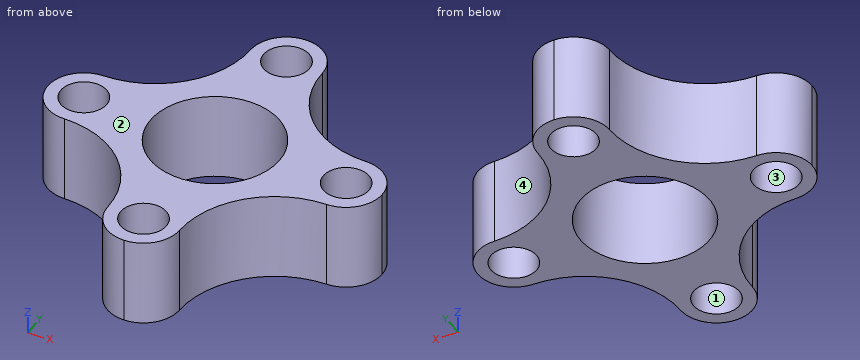
from build123d import *

# Parameters (mm, degrees)
AUFSATZ_LINEAR_AUSTRAGEN1_DEPTH = 10
SKIZZE2_R                       = 2.6
SCHNITT_LINEAR_AUSTRAGEN2_DEPTH = 10
SKIZZE3_R                       = 7.311453451
SCHNITT_LINEAR_AUSTRAGEN4_DEPTH = 10


with BuildPart() as part:
    # Skizze1 → Aufsatz-Linear austragen1 (new body)
    with BuildSketch(Plane.XY):
        with BuildLine():
            Line((0, 19.095775163), (0, 0))
            Line((0, 0), (19.095775163, 0))
            ThreePointArc((19.095775163, 0), (17.894912966, 2.899137803), (14.995775163, 4.1))
            ThreePointArc((14.995775163, 4.1), (7.291298659, 7.291298659), (4.1, 14.995775163))
            ThreePointArc((4.1, 14.995775163), (2.899137803, 17.894912966), (0, 19.095775163))
        make_face()
    extrude(amount=AUFSATZ_LINEAR_AUSTRAGEN1_DEPTH)

    # Spiegeln1: part across plane


with BuildPart() as part_1:
    add(part.part)
    add(part.part.mirror(Plane.ZX))

    # Spiegeln2: part across plane


with BuildPart() as part_2:
    add(part_1.part)
    add(part_1.part.mirror(Plane(origin=(0, 0, 0), x_dir=(0, 0, 1), z_dir=(1, 0, 0))))

    # Skizze2 → Schnitt-Linear austragen2 (cut)
    with BuildSketch(Plane.XY):
        with Locations((0, 14.995775163)):
            Circle(SKIZZE2_R)
        with Locations((14.995775163, 0)):
            Circle(SKIZZE2_R)
        with Locations((0, -14.995775163)):
            Circle(SKIZZE2_R)
        with Locations((-14.995775163, 0)):
            Circle(SKIZZE2_R)
    extrude(amount=SCHNITT_LINEAR_AUSTRAGEN2_DEPTH, mode=Mode.SUBTRACT)

    # Skizze3 → Schnitt-Linear austragen4 (cut)
    with BuildSketch(Plane.XY):
        Circle(SKIZZE3_R)
    extrude(amount=SCHNITT_LINEAR_AUSTRAGEN4_DEPTH, mode=Mode.SUBTRACT)


solid = part_2.part
Model file for the job. Use its own axes, mm. Face numbers are marked on the shaded views. Round coordinates to 2 decimals unless told otherwise and drop trailing zeros. Loops run counter-clockwise (first coordinate to the right, second up) from the corner with the lowest first, then second, coordinate; pieces in that order, holes last.
1. Drop flat-ended pins along their axis: P1, Ø1, axis at x = 2, z = 1.5, coming from the -Y side; P2, Ø2, axis at x = 8, z = 3.5, coming from the +Y side; P3, Ø1, axis at y = -2.5, z = 2, coming from the +X side. Give the stop position or say it passes through.
Check values:
P1: stops at y = -18.81
P2: stops at y = 7.59
P3: stops at x = 18.57
2. Band-saw the part on D-D, the plane y = 5.5. List the corners of the cut face in (x, z), and give its area (3 significant figures).
Check values:
outline: (-9.65, 0) - (-4.82, 0) - (-4.82, 10) - (-9.65, 10) - close; (4.82, 0) - (9.65, 0) - (9.65, 10) - (4.82, 10) - close
area: 96.7 mm2
3. Band-saw the part on B-B, the plane x = -14. List the corners of the cut face in (y, z), and give its area (3 significant figures).
Check values:
outline: (-4.15, 0) - (-2.4, 0) - (-2.4, 10) - (-4.15, 10) - close; (2.4, 0) - (4.15, 0) - (4.15, 10) - (2.4, 10) - close
area: 34.9 mm2
4. Band-saw the part on A-A, the plane z = 7.5. List the corners of the cut face in (x, y), and give its area (3 significant figures).
Check values:
outline: (-15, -4.1) arc R10.9 cw to (-4.1, -15) arc R4.1 ccw to (4.1, -15) arc R10.9 cw to (15, -4.1) arc R4.1 ccw to (15, 4.1) arc R10.9 cw to (4.1, 15) arc R4.1 ccw to (-4.1, 15) arc R10.9 cw to (-15, 4.1) arc R4.1 ccw to start; hole circle Ø5.2 at (-15, 0); hole circle Ø14.62 at (0, 0); hole circle Ø5.2 at (0, -15); hole circle Ø5.2 at (0, 15); hole circle Ø5.2 at (15, 0)
area: 379 mm2
5. Wall check: probe 1 along Y at (x, z) = (0, 2); probe 2 along Y at (x, z) = (-1, 1); probe 3 along Y at (x, z) = (-15, 8). Give the ranges that are in metal, low to high.
Check values:
probe 1: y = -19.1 to -17.6, -12.4 to -7.31, 7.31 to 12.4, 17.6 to 19.1
probe 2: y = -18.97 to -17.4, -12.6 to -7.24, 7.24 to 12.6, 17.4 to 18.97
probe 3: y = -4.1 to -2.6, 2.6 to 4.1
6. Band-saw the part on C-C, the plane x = -2. List the corners of the cut face in (y, z), and give its area (3 significant figures).
Check values:
outline: (-18.57, 0) - (-16.66, 0) - (-16.66, 10) - (-18.57, 10) - close; (-13.33, 0) - (-7.03, 0) - (-7.03, 10) - (-13.33, 10) - close; (7.03, 0) - (13.33, 0) - (13.33, 10) - (7.03, 10) - close; (16.66, 0) - (18.57, 0) - (18.57, 10) - (16.66, 10) - close
area: 164 mm2
7. Mould opens along Y. For the marked faces 1, 2, 3 and 4 say: +Y half, -Y half, draft (parallel to the pull), parting line (faces both ways), or undercut.
Check values:
face 1: undercut
face 2: draft
face 3: undercut
face 4: +Y half
